from build123d import *

# Parameters (mm, degrees)
EXTRUDE_DEPTH    = 10
EXTRUDE002_DEPTH = 2


with BuildPart() as extrude_body:
    # Extrude001 → Extrude (new body)
    with BuildSketch(Plane(origin=(-497.646447, 5, -142.853553), x_dir=(-1, 0, 0), z_dir=(0, -1, 0))):
        Polygon((0.353553, 4.646447), (-0.353553, 5.353553), (-0.353553, -4.646447), (0.353553, -5.353553), align=None)
        with BuildLine():
            Line((0.353553, -5.353553), (-0.353553, -4.646447))
            add(Edge.make_bspline(
                [(-0.353553, -4.646447), (-0.353553, -38.459309), (-8.155228, -72.64068)],
                knots=[13.797896, 13.797896, 13.797896, 81.348308, 81.348308, 81.348308], degree=2))
            Line((-8.155228, -72.64068), (-7.448121, -73.347786))
            add(Edge.make_bspline(
                [(0.353553, -5.353553), (0.353553, -39.166416), (-7.448121, -73.347786)],
                knots=[13.797896, 13.797896, 13.797896, 81.348308, 81.348308, 81.348308], degree=2))
        make_face()
        Polygon((-9.646447, 4.646447), (-10.353553, 5.353553), (-10.702548, -4.640355), (-9.995442, -5.347462), align=None)
        with BuildLine():
            Line((-9.995442, -5.347462), (-10.702548, -4.640355))
            add(Edge.make_bspline(
                [(-10.702548, -4.640355), (-11.917215, -39.423851), (-25.064253, -66.723956)],
                knots=[-74.623097, -74.623097, -74.623097, -14.39671, -14.39671, -14.39671], degree=2))
            Line((-25.064253, -66.723956), (-24.357146, -67.431063))
            add(Edge.make_bspline(
                [(-9.995442, -5.347462), (-11.210108, -40.130958), (-24.357146, -67.431063)],
                knots=[-74.623097, -74.623097, -74.623097, -14.39671, -14.39671, -14.39671], degree=2))
        make_face()
        Polygon((-19.646447, 4.646447), (-20.353553, 5.353553), (-21.398838, -4.591666), (-20.691731, -5.298772), align=None)
        with BuildLine():
            Line((-20.691731, -5.298772), (-21.398838, -4.591666))
            add(Edge.make_bspline(
                [(-21.398838, -4.591666), (-24.907666, -37.975933), (-40.232738, -57.192965)],
                knots=[-61.054819, -61.054819, -61.054819, -12.899631, -12.899631, -12.899631], degree=2))
            Line((-40.232738, -57.192965), (-39.525631, -57.900072))
            add(Edge.make_bspline(
                [(-20.691731, -5.298772), (-24.200559, -38.68304), (-39.525631, -57.900072)],
                knots=[-61.054819, -61.054819, -61.054819, -12.899631, -12.899631, -12.899631], degree=2))
        make_face()
        Polygon((-29.646447, 4.646447), (-30.353553, 5.353553), (-32.43267, -4.427923), (-31.725564, -5.135029), align=None)
        with BuildLine():
            Line((-31.725564, -5.135029), (-32.43267, -4.427923))
            add(Edge.make_bspline(
                [(-32.43267, -4.427923), (-38.517786, -33.05614), (-52.900072, -44.525631)],
                knots=[-43.534083, -43.534083, -43.534083, -7.65215, -7.65215, -7.65215], degree=2))
            Line((-52.900072, -44.525631), (-52.192965, -45.232738))
            add(Edge.make_bspline(
                [(-31.725564, -5.135029), (-37.810679, -33.763247), (-52.192965, -45.232738)],
                knots=[-43.534083, -43.534083, -43.534083, -7.65215, -7.65215, -7.65215], degree=2))
        make_face()
        Polygon((-39.646447, 4.646447), (-40.353553, 5.353553), (-43.773755, -4.043373), (-43.066648, -4.75048), align=None)
        with BuildLine():
            Line((-43.066648, -4.75048), (-43.773755, -4.043373))
            add(Edge.make_bspline(
                [(-43.773755, -4.043373), (-50.980104, -23.842655), (-62.431063, -29.357146)],
                knots=[-28.503789, -28.503789, -28.503789, -3.409115, -3.409115, -3.409115], degree=2))
            Line((-62.431063, -29.357146), (-61.723956, -30.064253))
            add(Edge.make_bspline(
                [(-43.066648, -4.75048), (-50.272997, -24.549761), (-61.723956, -30.064253)],
                knots=[-28.503789, -28.503789, -28.503789, -3.409115, -3.409115, -3.409115], degree=2))
        make_face()
        Polygon((-49.646447, 4.646447), (-50.353553, 5.353553), (-55.353553, -3.306701), (-54.646447, -4.013807), align=None)
        with BuildLine():
            Line((-54.646447, -4.013807), (-55.353553, -3.306701))
            add(Edge.make_bspline(
                [(-55.353553, -3.306701), (-59.460178, -10.419583), (-68.347786, -12.448121)],
                knots=[-5.337971, -5.337971, -5.337971, 10.390639, 10.390639, 10.390639], degree=2))
            Line((-68.347786, -12.448121), (-67.64068, -13.155228))
            add(Edge.make_bspline(
                [(-54.646447, -4.013807), (-58.753071, -11.126689), (-67.64068, -13.155228)],
                knots=[-5.337971, -5.337971, -5.337971, 10.390639, 10.390639, 10.390639], degree=2))
        make_face()
    extrude(amount=EXTRUDE_DEPTH)


with BuildPart() as cut:
    # Sketch → Extrude002 (new body)
    with BuildSketch(Plane.XZ):
        Polygon((-507.364975, -157.790507), (-437.364975, -157.790507), (-437.364975, -147.790507), (492.635025, -147.790507), (492.635025, 79.992619), (502.635025, 79.992619), (502.635025, 149.992619), (492.635025, 149.992619), (492.635025, 153.209493), (422.635025, 153.209493), (422.635025, 152.209493), (-507.364975, 152.209493), (-507.364975, -77.790507), (-508.364975, -77.790507), (-508.364975, -147.790507), (-507.364975, -147.790507), align=None)
    extrude(amount=EXTRUDE002_DEPTH)

    # Cut: cut Extrude body
    add(extrude_body.part, mode=Mode.SUBTRACT)


solid = cut.part
Build history of the part. All positions in model axes, mm. Round coordinates to 2 decimals unless told otherwise and drop trailing zeros. Write each loop counter-clockwise with the first axis right and the second up, starting at its lowest first coordinate (ties: lowest second). Pieces come first, ordered by that corner, then holes. Notation, with made-up numbers: M 16.25,-6 L 73.25,-6 A26 ccw 73.25,30 Z; hole C -19.5,-1 d10. An arc over 180 degrees is marked long. Use CSV: the item, a comma, the result in double quotes.
1. Flat gauge pins, fed straight in: pin 1 (1 mm diameter, centred on y = -1, z = 151, fed in from +X) (3 decimals); pin 2 (1 mm diameter, centred on y = -1.5, z = 44.5, fed in from -X) (3 decimals); pin 3 (0.6 mm diameter, centred on y = -1, z = -153, fed in from +X) (3 decimals). Where does each tip first touch, or does it go through?
Reply:
pin 1,"stops at x = 492.635"
pin 2,"stops at x = -507.365"
pin 3,"stops at x = -437.365"
2. Wall check: probe 1 along X at (y, z) = (-0.75, -106.5); probe 2 along X at (y, z) = (-1.2, -124.5); probe 3 along Z at (x, y) = (-15.5, -0.3). Give the ranges that are in metal, low to high. Write a range as from..to.
Reply:
probe 1,"x = -508.36..-496.37, -495.59..-483.88, -483.02..-470.05, -469.07..-453.66, -452.45..492.64"
probe 2,"x = -508.36..-497.71, -496.97..-486.75, -485.97..-475.03, -474.18..-462.37, -461.42..-448.1, -446.94..492.64"
probe 3,"z = -147.79..152.21"
3. Saw through at B-B (x = -305). Give the cut face in (y, z), plus the area to 3 significant figures.
Reply:
outline,"M -2,-147.79 L 0,-147.79 L 0,152.21 L -2,152.21 Z"
area,"600 mm²"
4. Saw through at A-A (y = -0.95). State how many separate pieces and enclosed holes the cut face has, plus the area to 3 significant figures.
Reply:
separate pieces,"1"
enclosed holes,"6"
area,"301,000 mm²"
